Input: part model. Units: mm. Frame: model coordinates. Round coordinates to 2 decimals unless told otherwise and drop trailing zeros. Loops run counter-clockwise (first coordinate to the right, second up) from the corner with the lowest first, then second, coordinate; pieces in that order, holes last. Notation, with made-up numbers: M 50.5,-16 L 80.5,-16 A19 cw 80.5,12 Z; hole C 26.25,-9.5 d1. An arc over 180 degrees is marked long. Use one line per item in the form item = value. Start each with the question number.
Q1. Section query B-B, the plane x = 45. Output: boundary loops of the cut face in (y, z).
Q2. Mould query, pull axis X, two halves, no side actions, for faces 1 (the flat face through (-1, 4, 0)), 2 (the cylindrical face through (-26.2, -9.1, 1)), 3 (the cylindrical face through (-25.208, 19.086, 1.014)), 4 (the flat face through (50, 3, 1)). Classes: pulls with the +X half, pulls with the -X half, needs draft (parallel to the pull), parting line crosses it, or undercut.
Q3. First-contact query: P1, Ø1.9, axis at x = -25, y = -10.16, coming from the +Z side; P2, Ø10, axis at x = -35, y = -6, coming from the -Z side. Flat tips, straight axial feed; report the tip coordinate or a pass-through.
Q4. Ray query, line 1 along Y through (x, z) = (25, 0.5); line 2 along X through (y, z) = (-7.5, 0.55); line 3 along X through (y, z) = (-11, 0.15). Return the intervals inside material, ascending.
Q5. Section query C-C, the plane z = 1.05. State how many separate pieces and enclosed holes the cut face has, and give its area (3 significant figures).
Q6. Section query D-D, the plane x = 15.75. Output: boundary loops of the cut face in (y, z).
Q7. Section query A-A, the plane x = 0. Output: boundary loops of the cut face in (y, z).
```python
from build123d import *

# Parameters (mm, degrees)
SKETCH_1_W          = 100
SKETCH_1_H          = 50
SKETCH_1_R          = 1.6
EXTRUDE_1_DEPTH     = 2
SKETCH_3_R          = 6
CUT_EXTRUDE_2_DEPTH = 2
SKETCH_4_R          = 1.6
CUT_EXTRUDE_3_DEPTH = 2
CUT_EXTRUDE_7_DEPTH = 3
SKETCH_6_W          = 100
SKETCH_6_H          = 2
CUT_EXTRUDE_8_DEPTH = 7.34
SKETCH_7_R          = 1.6
CUT_EXTRUDE_9_DEPTH = 10


with BuildPart() as part:
    # ｽｹｯﾁ1 → ﾎﾞｽ - 押し出し1 (new body)
    with BuildSketch(Plane.XY):
        Rectangle(SKETCH_1_W, SKETCH_1_H)
        with Locations((-15.75, 6.5)):
            Circle(SKETCH_1_R, mode=Mode.SUBTRACT)
        with Locations((15.75, 6.5)):
            Circle(SKETCH_1_R, mode=Mode.SUBTRACT)
    extrude(amount=EXTRUDE_1_DEPTH)

    # ｽｹｯﾁ3 → ｶｯﾄ - 押し出し2 (cut)
    with BuildSketch(Plane.XY.offset(2)):
        with Locations((0, 13.5)):
            Circle(SKETCH_3_R)
    extrude(amount=-CUT_EXTRUDE_2_DEPTH, mode=Mode.SUBTRACT)

    # ｽｹｯﾁ4 → ｶｯﾄ - 押し出し3 (cut)
    with BuildSketch(Plane.XY.offset(2)):
        with Locations((-7.875, 20.13990011)):
            Circle(SKETCH_4_R)
        with Locations((7.875, 20.13990011)):
            Circle(SKETCH_4_R)
        with Locations((-7.875, -7.13990011)):
            Circle(SKETCH_4_R)
        with Locations((7.875, -7.13990011)):
            Circle(SKETCH_4_R)
    extrude(amount=-CUT_EXTRUDE_3_DEPTH, mode=Mode.SUBTRACT)

    # ｽｹｯﾁ5 → ｶｯﾄ - 押し出し7 (cut, through all)
    with BuildSketch(Plane.XY.offset(2)):
        with BuildLine():
            ThreePointArc((-46.6, -10.16), (-45, -11.76), (-43.4, -10.16))
            Line((-43.4, -10.16), (-45, -10.16))
            Line((-45, -10.16), (-46.6, -10.16))
        make_face()
        with BuildLine():
            Line((-45, -10.16), (-43.4, -10.16))
            ThreePointArc((-43.4, -10.16), (-45, -8.56), (-46.6, -10.16))
            Line((-46.6, -10.16), (-45, -10.16))
        make_face()
        with BuildLine():
            ThreePointArc((-26.6, -10.16), (-25, -11.76), (-23.4, -10.16))
            Line((-23.4, -10.16), (-25, -10.16))
            Line((-25, -10.16), (-26.6, -10.16))
        make_face()
        with BuildLine():
            Line((-25, -10.16), (-23.4, -10.16))
            ThreePointArc((-23.4, -10.16), (-25, -8.56), (-26.6, -10.16))
            Line((-26.6, -10.16), (-25, -10.16))
        make_face()
        with BuildLine():
            ThreePointArc((46.6, -10.16), (45, -8.56), (43.4, -10.16))
            Line((43.4, -10.16), (45, -10.16))
            Line((45, -10.16), (46.6, -10.16))
        make_face()
        with BuildLine():
            Line((45, -10.16), (43.4, -10.16))
            ThreePointArc((43.4, -10.16), (45, -11.76), (46.6, -10.16))
            Line((46.6, -10.16), (45, -10.16))
        make_face()
        with BuildLine():
            ThreePointArc((26.6, -10.16), (25, -8.56), (23.4, -10.16))
            Line((23.4, -10.16), (25, -10.16))
            Line((25, -10.16), (26.6, -10.16))
        make_face()
        with BuildLine():
            Line((25, -10.16), (23.4, -10.16))
            ThreePointArc((23.4, -10.16), (25, -11.76), (26.6, -10.16))
            Line((26.6, -10.16), (25, -10.16))
        make_face()
    extrude(amount=-CUT_EXTRUDE_7_DEPTH, mode=Mode.SUBTRACT)

    # ｽｹｯﾁ6 → ｶｯﾄ - 押し出し8 (cut)
    with BuildSketch(Plane.XZ.offset(25)):
        with Locations((0, 1)):
            Rectangle(SKETCH_6_W, SKETCH_6_H)
    extrude(amount=-CUT_EXTRUDE_8_DEPTH, mode=Mode.SUBTRACT)

    # ｽｹｯﾁ7 → ｶｯﾄ - 押し出し9 (cut)
    with BuildSketch(Plane.XY.offset(2)):
        with Locations((-45, 17.5)):
            Circle(SKETCH_7_R)
        with Locations((-25, 17.5)):
            Circle(SKETCH_7_R)
        with Locations((45, 17.5)):
            Circle(SKETCH_7_R)
        with Locations((25, 17.5)):
            Circle(SKETCH_7_R)
    extrude(amount=-CUT_EXTRUDE_9_DEPTH, mode=Mode.SUBTRACT)


solid = part.part
```
Results found:
q1.outline = M -17.66,0 L -11.76,0 L -11.76,2 L -17.66,2 Z; M -8.56,0 L 15.9,0 L 15.9,2 L -8.56,2 Z; M 19.1,0 L 25,0 L 25,2 L 19.1,2 Z
q2.face_1 = needs draft
q2.face_2 = undercut
q2.face_3 = undercut
q2.face_4 = pulls with the +X half
q3.P1 = through
q3.P2 = 0
q4.line_1 = -17.66 to -11.76, -8.56 to 15.9, 19.1 to 25
q4.line_2 = -50 to -9.43, -6.32 to 6.32, 9.43 to 50
q4.line_3 = -50 to -46.36, -43.64 to -26.36, -23.64 to 23.64, 26.36 to 43.64, 46.36 to 50
q5.separate_pieces = 1
q5.enclosed_holes = 15
q5.area = 4,040 mm²
q6.outline = M -17.66,0 L 4.9,0 L 4.9,2 L -17.66,2 Z; M 8.1,0 L 25,0 L 25,2 L 8.1,2 Z
q7.outline = M -17.66,0 L 7.5,0 L 7.5,2 L -17.66,2 Z; M 19.5,0 L 25,0 L 25,2 L 19.5,2 Z
